Work out the finished part from the listing and answer in its coordinate system (mm). A direction names the side the tool comes from. Give positions to 0.01 mm unless a question says otherwise; leave off trailing zeros. Order: outer loops, then holes, each group sorted by start corner. A loop starts at its lowest first (then second) coordinate and runs counter-clockwise, first axis right, second up.
```python
from build123d import *

# Parameters (mm, degrees)
SKETCH_1_W          = 27.85
SKETCH_1_H          = 27.85
SKETCH_1_R          = 1.25
SKETCH_1_R_2        = 3.75
EXTRUDE_1_DEPTH     = 7
SKETCH_1_4_R        = 1.25
CUT_EXTRUDE_1_DEPTH = 1.8
CHAMFER_1_SIZE      = 1
FILLET_1_R          = 2
SKETCH_3_R          = 6.5
CUT_EXTRUDE_2_DEPTH = 5
CHAMFER_2_SIZE      = 0.2


with BuildPart() as part:
    # Sketch 1 → Extrude 1 (new body)
    with BuildSketch(Plane(origin=(0, 0, 0), x_dir=(1, 0, 0), z_dir=(0, 1, 0))):
        Rectangle(SKETCH_1_W, SKETCH_1_H)
        with Locations((-11.5, 11.5)):
            Circle(SKETCH_1_R, mode=Mode.SUBTRACT)
        with Locations((11.5, 11.5)):
            Circle(SKETCH_1_R, mode=Mode.SUBTRACT)
        with Locations((-11.5, -11.5)):
            Circle(SKETCH_1_R, mode=Mode.SUBTRACT)
        with Locations((11.5, -11.5)):
            Circle(SKETCH_1_R, mode=Mode.SUBTRACT)
        Circle(SKETCH_1_R_2, mode=Mode.SUBTRACT)
    extrude(amount=EXTRUDE_1_DEPTH)

    # Sketch 1_4 → Cut-Extrude 1 (cut)
    with BuildSketch(Plane(origin=(0, 0, 0), x_dir=(1, 0, 0), z_dir=(0, 1, 0))):
        with BuildLine():
            Line((-9.144874717, 13.925), (-13.925, 13.925))
            Line((-13.925, 13.925), (-13.925, 9.144874717))
            Line((-13.925, 9.144874717), (-11.144874717, 9.144874717))
            ThreePointArc((-11.144874717, 9.144874717), (-9.730661155, 9.730661155), (-9.144874717, 11.144874717))
            Line((-9.144874717, 11.144874717), (-9.144874717, 13.925))
        make_face()
        with Locations((-11.5, 11.5)):
            Circle(SKETCH_1_4_R, mode=Mode.SUBTRACT)
        with BuildLine():
            Line((13.925, 13.925), (9.144874717, 13.925))
            Line((9.144874717, 13.925), (9.144874717, 11.144874717))
            ThreePointArc((9.144874717, 11.144874717), (9.730661155, 9.730661155), (11.144874717, 9.144874717))
            Line((11.144874717, 9.144874717), (13.925, 9.144874717))
            Line((13.925, 9.144874717), (13.925, 13.925))
        make_face()
        with Locations((11.5, 11.5)):
            Circle(SKETCH_1_4_R, mode=Mode.SUBTRACT)
        with BuildLine():
            Line((-11.144874717, -9.144874717), (-13.925, -9.144874717))
            Line((-13.925, -9.144874717), (-13.925, -13.925))
            Line((-13.925, -13.925), (-9.144874717, -13.925))
            Line((-9.144874717, -13.925), (-9.144874717, -11.144874717))
            ThreePointArc((-9.144874717, -11.144874717), (-9.730661155, -9.730661155), (-11.144874717, -9.144874717))
        make_face()
        with Locations((-11.5, -11.5)):
            Circle(SKETCH_1_4_R, mode=Mode.SUBTRACT)
        with BuildLine():
            Line((13.925, -13.925), (13.925, -9.144874717))
            Line((13.925, -9.144874717), (11.144874717, -9.144874717))
            ThreePointArc((11.144874717, -9.144874717), (9.730661155, -9.730661155), (9.144874717, -11.144874717))
            Line((9.144874717, -11.144874717), (9.144874717, -13.925))
            Line((9.144874717, -13.925), (13.925, -13.925))
        make_face()
        with Locations((11.5, -11.5)):
            Circle(SKETCH_1_4_R, mode=Mode.SUBTRACT)
    extrude(amount=CUT_EXTRUDE_1_DEPTH, mode=Mode.SUBTRACT)

    # Chamfer 1
    chamfer_1_edges = [part.edges().sort_by_distance(p)[0] for p in [
        (-9.144874717, 0, 12.534937359),
        (-9.730661155, 0, 9.730661155),
        (-12.534937359, 0, 9.144874717),
        (12.534937359, 0, 9.144874717),
        (9.730661155, 0, 9.730661155),
        (9.144874717, 0, 12.534937359),
        (9.144874717, 0, -12.534937359),
        (9.730661155, 0, -9.730661155),
        (12.534937359, 0, -9.144874717),
        (-12.534937359, 0, -9.144874717),
        (-9.730661155, 0, -9.730661155),
        (-9.144874717, 0, -12.534937359),
    ]]
    chamfer(chamfer_1_edges, length=CHAMFER_1_SIZE)

    # Fillet 1
    fillet_1_edges = [part.edges().sort_by_distance(p)[0] for p in [
        (13.925, 4.4, -13.925),
        (13.925, 4.4, 13.925),
        (-13.925, 4.4, 13.925),
        (-13.925, 4.4, -13.925),
    ]]
    fillet(fillet_1_edges, radius=FILLET_1_R)

    # Sketch 3 → Cut-Extrude 2 (cut)
    with BuildSketch(Plane(origin=(0, 7, 0), x_dir=(1, 0, 0), z_dir=(0, 1, 0))):
        Circle(SKETCH_3_R)
    extrude(amount=-CUT_EXTRUDE_2_DEPTH, mode=Mode.SUBTRACT)

    # Chamfer 2
    chamfer_2_edges = [part.edges().sort_by_distance(p)[0] for p in [
        (-3.75, 0, 0),
        (-3.75, 2, 0),
        (-6.5, 7, 0),
    ]]
    chamfer(chamfer_2_edges, length=CHAMFER_2_SIZE)


solid = part.part
```
1. The part is cut by section D-D (y = 5.25). Write down the section's boundary in (x, z) (3 decimals).
Findings below:
outline: (-13.925, -11.925) arc R2 ccw to (-11.925, -13.925) - (11.925, -13.925) arc R2 ccw to (13.925, -11.925) - (13.925, 11.925) arc R2 ccw to (11.925, 13.925) - (-11.925, 13.925) arc R2 ccw to (-13.925, 11.925) - close; hole circle Ø2.5 at (-11.5, -11.5); hole circle Ø2.5 at (-11.5, 11.5); hole circle Ø13 at (0, 0); hole circle Ø2.5 at (11.5, -11.5); hole circle Ø2.5 at (11.5, 11.5)
2. Given P1, Ø5.5, axis at x = -12, z = -11, coming from the -Y side; P2, Ø1.5, axis at x = 11.5, z = 11.5, coming from the +Y side; P3, Ø4, axis at x = -12, z = 11.5, coming from the -Y side; P4, Ø12, axis at x = 2.5, z = 1, coming from the -Y side, each flat-ended and moving along its own axis, determine where each tip first touches the part or whether it passes through.
Findings below:
P1: stops at y = 0.11
P2: passes through
P3: stops at y = 1.8
P4: stops at y = 0
3. The part is cut by section C-C (z = -11.5). Write down the section's boundary in (x, y) (3 decimals).
Findings below:
outline: (-13.925, 1.8) - (-12.75, 1.8) - (-12.75, 7) - (-13.925, 7) - close; (-10.25, 1.8) - (-9.145, 1.8) - (-9.145, 1) - (-8.145, 0) - (8.145, 0) - (9.145, 1) - (9.145, 1.8) - (10.25, 1.8) - (10.25, 7) - (-10.25, 7) - close; (12.75, 1.8) - (13.925, 1.8) - (13.925, 7) - (12.75, 7) - close
4. Straight lines are drawn through the part: probe 1 along X at (y, z) = (5.1, 11.5) (3 decimals); probe 2 along X at (y, z) = (0.75, 0) (3 decimals). For each, find the intervals that lie inside material, in ascending order.
Findings below:
probe 1: x = -13.925 to -12.75, -10.25 to 10.25, 12.75 to 13.925
probe 2: x = -13.925 to -3.75, 3.75 to 13.925
5. The part is cut by section A-A (z = 0). Write down the section's boundary in (x, y) (3 decimals), then the cut area to 3 significant figures.
Findings below:
outline: (-13.925, 0) - (-3.95, 0) - (-3.75, 0.2) - (-3.75, 1.8) - (-3.95, 2) - (-6.5, 2) - (-6.5, 6.8) - (-6.7, 7) - (-13.925, 7) - close; (3.75, 0.2) - (3.95, 0) - (13.925, 0) - (13.925, 7) - (6.7, 7) - (6.5, 6.8) - (6.5, 2) - (3.95, 2) - (3.75, 1.8) - close
area: 115 mm2
6. Which of the six approach directions +Z, -Z, +X, -X, +Y, -Y give full straight-line access (tool end or side, diameter ignored) to faces 5 (the face through (10, 1.8, 10)), 6 (the face through (12.5, 1.4, -9.145)), 7 (the face through (-12, 1.8, -13))?
Findings below:
face 5: +Z, +X, -Y
face 6: -Z, +X, -Y
face 7: -Z, -X, -Y
7. The part is cut by section B-B (x = -11.5). Write down the section's boundary in (y, z) (3 decimals), then the cut area to 3 significant figures.
Findings below:
outline: (0, -8.145) - (1, -9.145) - (1.8, -9.145) - (1.8, -10.25) - (7, -10.25) - (7, 10.25) - (1.8, 10.25) - (1.8, 9.145) - (1, 9.145) - (0, 8.145) - close; (1.8, -13.925) - (7, -13.925) - (7, -12.75) - (1.8, -12.75) - close; (1.8, 12.75) - (7, 12.75) - (7, 13.925) - (1.8, 13.925) - close
area: 151 mm2
8. The mould has two halves that part along Z. Classify faces 1 (the face through (12.6, 1.4, 9.145)), 2 (the face through (-12.6, 1.4, -9.145)), 3 (the face through (-8.652, 0.507, 12.554)), 4 (the face through (-12.421, 4.364, -12.345)): pulls with the +Z half, pulls with the -Z half, needs draft (parallel to the pull), parting line crosses it, or undercut.
Findings below:
face 1: pulls with the +Z half
face 2: pulls with the -Z half
face 3: needs draft
face 4: undercut
